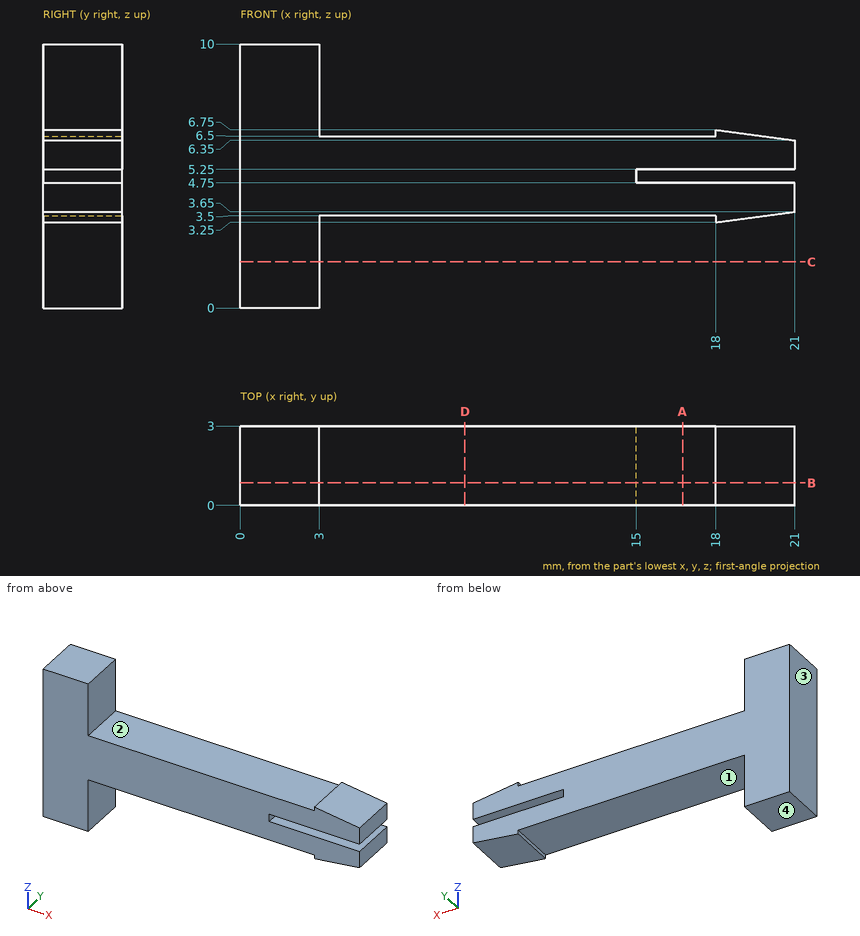
Geometry: see drawing. Coordinates: mm, zero at the bounding-box minimum. Give positions to 0.01 mm unless a question says otherwise; leave off trailing zeros. Write each loop counter-clockwise with the first axis right and the second up, starting at its lowest first coordinate (ties: lowest second). Pieces come first, ordered by that corner, then holes. Notation, with made-up numbers: M 34,7 L 50,7 A35 ccw 50,39 Z; hole C 36,78.25 d2. An arc over 180 degrees is marked long. Return JSON: item names as keys, results as strings. Group by question number.
1) Cut plane D-D, the plane x = 8.5. Output: boundary loops of the cut face in (y, z).
2) Cut plane A-A, the plane x = 16.75. Output: boundary loops of the cut face in (y, z), then the cut area to 3 significant figures.
3) Draft query along X for the marked faces 1, 2, 3 and 4. Return one class per face: released by +X, released by -X, zero draft, split by the parting line, or undercut.
4) Cut plane C-C, the plane z = 1.75. Output: boundary loops of the cut face in (x, y), then the cut area to 3 significant figures.
5) First-contact query: pin 1 Ø1.5 at (x, y) = (17, 1.5) entering from +Z; pin 2 Ø0.9 at (x, y) = (18, 1) entering from -Z; pin 3 Ø0.9 at (y, z) = (1, 8) entering from +X. Flat tips, straight axial feed; report the tip coordinate or a pass-through.
6) Cut plane B-B, the plane y = 0.85. Output: boundary loops of the cut face in (x, z).
7) Ray query, L1, parallel to Z at x = 17.5, y = 2.4; L2, parallel to Z at x = 3.75, y = 1.2; L3, parallel to X at y = 2.3, z = 9. Return the intervals inside material, ascending.
Data:
{
 "1": {"outline": "M 0,3.5 L 3,3.5 L 3,6.5 L 0,6.5 Z"},
 "2": {"outline": "M 0,3.5 L 3,3.5 L 3,4.75 L 0,4.75 Z; M 0,5.25 L 3,5.25 L 3,6.5 L 0,6.5 Z", "area": "7.50 mm²"},
 "3": {"face 1": "undercut", "face 2": "undercut", "face 3": "released by -X", "face 4": "zero draft"},
 "4": {"outline": "M 0,0 L 3,0 L 3,3 L 0,3 Z", "area": "9.00 mm²"},
 "5": {"pin 1": "stops at z = 6.5", "pin 2": "stops at z = 3.25", "pin 3": "stops at x = 3"},
 "6": {"outline": "M 0,0 L 3,0 L 3,3.5 L 18,3.5 L 18,3.25 L 21,3.65 L 21,4.75 L 15,4.75 L 15,5.25 L 21,5.25 L 21,6.35 L 18,6.75 L 18,6.5 L 3,6.5 L 3,10 L 0,10 Z"},
 "7": {"L1": "z = 3.5 to 4.75, 5.25 to 6.5", "L2": "z = 3.5 to 6.5", "L3": "x = 0 to 3"}
}
